Geometry check sheet. Reference: the model listing, model coordinates, mm. Face numbers are marked on the shaded views. A direction names the side the tool comes from. Round coordinates to 2 decimals unless told otherwise and drop trailing zeros. Order: outer loops, then holes, each group sorted by start corner. A loop starts at its lowest first (then second) coordinate and runs counter-clockwise, first axis right, second up.
(1) Sectioned sample at A-A (y = -20). Record the boundary of the cut face in (x, z), plus the area to 3 significant figures.
(2) Set-up check for the marked faces 1, 2 and 3: record each of +Z, -Z, +X, -X, +Y, -Y from which the full face is reachable in a straight line by a thin tool's end or side.
(3) Sectioned sample at C-C (z = 6.5). Record the boundary of the cut face in (x, y), plus the area to 3 significant figures.
(4) Material ranges on line 1 along Z through (x, y) = (15, -30); line 2 along X through (y, z) = (-3, 9.5); line 3 along X through (y, z) = (-27.5, 0.5), recorded low to high.
(5) Sectioned sample at D-D (y = 1.85). Record the boundary of the cut face in (x, z).
(6) Go/stop test with flat-tipped pins: pin 1 (3.5 mm diameter, centred on x = 28, z = 9, fed in from -Y); pin 2 (2.5 mm diameter, centred on x = -15, z = 6.5, fed in from +Y); pin 3 (1.5 mm diameter, centred on x = 14.5, z = -7, fed in from -Y); pin 4 (2 mm diameter, centred on x = 24, y = -10.5, fed in from +Z). Record where each tip stops, or that it passes through.
(7) Sectioned sample at B-B (x = -5). Record the boundary of the cut face in (y, z), plus the area to 4 significant figures.
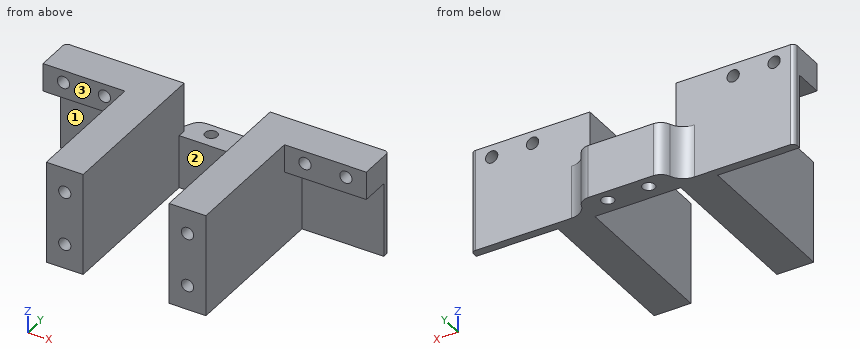
from build123d import *

# Parameters (mm, degrees)
SKETCH_W        = 79
SKETCH_H        = 25
PAD_DEPTH       = 2
SKETCH001_W     = 21
SKETCH001_H     = 25
PAD001_DEPTH    = 4.85
SKETCH002_R     = 1.5
POCKET_DEPTH    = 25.001
SKETCH003_W     = 21
SKETCH003_H     = 12
POCKET001_DEPTH = 10
PAD002_DEPTH    = 6.85
SKETCH005_W     = 9
SKETCH005_H     = 38.5
PAD003_DEPTH    = 18.15
SKETCH006_R     = 1.5
POCKET002_DEPTH = 10
SKETCH007_R     = 1.5
POCKET003_DEPTH = 22
FILLET_R        = 4.5
FILLET001_R     = 3
FILLET002_R     = 1


with BuildPart() as part:
    # Sketch → Pad (new body)
    with BuildSketch(Plane.XZ):
        Rectangle(SKETCH_W, SKETCH_H)
    extrude(amount=PAD_DEPTH)

    # Sketch001 (on Face5 of Pad) → Pad001 (join)
    with BuildSketch(Plane(origin=(0, 0, 0), x_dir=(1, 0, 0), z_dir=(0, 1, 0))):
        Rectangle(SKETCH001_W, SKETCH001_H)
    extrude(amount=PAD001_DEPTH)

    # Sketch002 (on Face5 of Pad001) → Pocket (cut, through all)
    with BuildSketch(Plane(origin=(0, 0, 12.5), x_dir=(-1, 0, 0), z_dir=(0, 0, 1))):
        with Locations((-5, -1.85)):
            Circle(SKETCH002_R)
        with Locations((5, -1.85)):
            Circle(SKETCH002_R)
    extrude(amount=-POCKET_DEPTH, mode=Mode.SUBTRACT)

    # Sketch003 (on Face11 of Pocket) → Pocket001 (cut)
    with BuildSketch(Plane(origin=(0, 4.85, 0), x_dir=(1, 0, 0), z_dir=(0, 1, 0))):
        with Locations((0, -6.5)):
            Rectangle(SKETCH003_W, SKETCH003_H)
    extrude(amount=-POCKET001_DEPTH, mode=Mode.SUBTRACT)

    # Sketch004 (on DatumPlane) → Pad002 (join)
    with BuildSketch(Plane(origin=(0, -12.5, 12.5), x_dir=(-1, 0, 0), z_dir=(0, 0, 1))):
        Polygon((39.5, -10.5), (10.5, -10.5), (10.5, 28), (19.5, 28), (19.5, -3.5), (39.5, -3.5), align=None)
        Polygon((-10.5, -10.5), (-10.5, 28), (-19.5, 28), (-19.5, -3.5), (-39.5, -3.5), (-39.5, -10.5), align=None)
    extrude(amount=-PAD002_DEPTH)

    # Sketch005 (on Face21 of Pad002) → Pad003 (join)
    with BuildSketch(Plane(origin=(0, 0, 5.65), x_dir=(1, 0, 0), z_dir=(0, 0, -1))):
        with Locations((-15, 21.25)):
            Rectangle(SKETCH005_W, SKETCH005_H)
        with Locations((15, 21.25)):
            Rectangle(SKETCH005_W, SKETCH005_H)
    extrude(amount=PAD003_DEPTH)

    # Sketch006 (on Face17 of Pad003) → Pocket002 (cut)
    with BuildSketch(Plane(origin=(0, 0, 0), x_dir=(1, 0, 0), z_dir=(0, 1, 0))):
        with Locations((-34.5, -9.5)):
            Circle(SKETCH006_R)
        with Locations((-24.5, -9.5)):
            Circle(SKETCH006_R)
        with Locations((24.5, -9.5)):
            Circle(SKETCH006_R)
        with Locations((34.5, -9.5)):
            Circle(SKETCH006_R)
    extrude(amount=-POCKET002_DEPTH, mode=Mode.SUBTRACT)

    # Sketch007 (on Face26 of Pocket002) → Pocket003 (cut)
    with BuildSketch(Plane.XZ.offset(40.5)):
        with Locations((-15, 6.5)):
            Circle(SKETCH007_R)
        with Locations((-15, -6.5)):
            Circle(SKETCH007_R)
        with Locations((15, 6.5)):
            Circle(SKETCH007_R)
        with Locations((15, -6.5)):
            Circle(SKETCH007_R)
    extrude(amount=-POCKET003_DEPTH, mode=Mode.SUBTRACT)

    # Fillet
    fillet_edges = [part.edges().sort_by_distance(p)[0] for p in [
        (10.5, 0, -6),
        (-10.5, 0, -6),
    ]]
    fillet(fillet_edges, radius=FILLET_R)

    # Fillet001
    fillet001_edges = [part.edges().sort_by_distance(p)[0] for p in [
        (10.5, 4.85, -6),
        (-10.5, 4.85, -6),
    ]]
    fillet(fillet001_edges, radius=FILLET001_R)

    # Fillet002
    fillet002_edges = [part.edges().sort_by_distance(p)[0] for p in [
        (39.5, 0, 0),
        (-39.5, 0, 0),
    ]]
    fillet(fillet002_edges, radius=FILLET002_R)


solid = part.part
Answer below:
1. outline: (-19.5, -12.5) - (-10.5, -12.5) - (-10.5, 12.5) - (-19.5, 12.5) - close; (10.5, -12.5) - (19.5, -12.5) - (19.5, 12.5) - (10.5, 12.5) - close; hole circle Ø3 at (-15, -6.5); hole circle Ø3 at (-15, 6.5); hole circle Ø3 at (15, -6.5); hole circle Ø3 at (15, 6.5)
1. area: 422 mm2
2. face 1: -Z, -X, -Y
2. face 2: +Z, -Z, -Y
2. face 3: +Z, -Z, -X, -Y
3. outline: (-39.5, -9) - (-19.5, -9) - (-19.5, -40.5) - (-16.5, -40.5) - (-16.5, -18.5) - (-13.5, -18.5) - (-13.5, -40.5) - (-10.5, -40.5) - (-10.5, 0) - (-38.5, 0) arc R1 ccw to (-39.5, -1) - close; (10.5, -40.5) - (13.5, -40.5) - (13.5, -18.5) - (16.5, -18.5) - (16.5, -40.5) - (19.5, -40.5) - (19.5, -9) - (39.5, -9) - (39.5, -1) arc R1 ccw to (38.5, 0) - (10.5, 0) - close
3. area: 957 mm2
4. line 1: z = -12.5 to -8, -5 to 5, 8 to 12.5
4. line 2: x = -39.5 to -36, -33 to -26, -23 to -10.5, 10.5 to 23, 26 to 33, 36 to 39.5
4. line 3: x = -19.5 to -10.5, 10.5 to 19.5
5. outline: (-11.36, -12.5) - (-6.5, -12.5) - (-6.5, 0.5) - (-11.36, 0.5) - close; (-3.5, -12.5) - (3.5, -12.5) - (3.5, 0.5) - (-3.5, 0.5) - close; (6.5, -12.5) - (11.36, -12.5) - (11.36, 0.5) - (6.5, 0.5) - close
6. pin 1: stops at y = -9
6. pin 2: stops at y = 0
6. pin 3: stops at y = -18.5
6. pin 4: passes through
7. outline: (-2, -12.5) - (0.35, -12.5) - (0.35, 0.5) - (-2, 0.5) - close; (3.35, -12.5) - (4.85, -12.5) - (4.85, 0.5) - (3.35, 0.5) - close
7. area: 50.05 mm2
